CAD build for the part. Positions are in the model's coordinates, mm. Face numbers are marked on the shaded views. A direction names the side the tool comes from. Coordinates: 2 decimals unless noted, no trailing zeros. Order: outer loops, then holes, each group sorted by start corner. A loop starts at its lowest first (then second) coordinate and runs counter-clockwise, first axis right, second up. Notation, with made-up numbers: M 63,-36 L 118,-36 A20 ccw 118,-26 Z; hole C 70.5,30 d6. An arc over 180 degrees is marked long. One line per item, written item: value.
from build123d import *

# Parameters (mm, degrees)
SKETCH1_W           = 41.91
SKETCH1_H           = 41.91
SKETCH1_R           = 1.64973
SKETCH1_R_2         = 12.7
BOSS_EXTRUDE1_DEPTH = 10.795
SKETCH2_R           = 62.565718238
SKETCH2_R_2         = 27.7876
CUT_EXTRUDE1_DEPTH  = 61.244736077
SKETCH3_R           = 19.84375
CUT_EXTRUDE2_DEPTH  = 7.62


with BuildPart() as part:
    # Sketch1 → Boss-Extrude1 (new body)
    with BuildSketch(Plane.XY):
        with Locations((20.955, 20.955)):
            Rectangle(SKETCH1_W, SKETCH1_H)
        with Locations((37.460710751, 37.460710751)):
            Circle(SKETCH1_R, mode=Mode.SUBTRACT)
        with Locations((37.460710751, 4.449289249)):
            Circle(SKETCH1_R, mode=Mode.SUBTRACT)
        with Locations((4.449289249, 4.449289249)):
            Circle(SKETCH1_R, mode=Mode.SUBTRACT)
        with Locations((4.449289249, 37.460710751)):
            Circle(SKETCH1_R, mode=Mode.SUBTRACT)
        with Locations((20.955, 20.955)):
            Circle(SKETCH1_R_2, mode=Mode.SUBTRACT)
    extrude(amount=BOSS_EXTRUDE1_DEPTH)

    # Sketch2 → Cut-Extrude1 (cut, through all)
    with BuildSketch(Plane.XY.offset(10.795)):
        with Locations((20.955, 20.955)):
            Circle(SKETCH2_R)
        with Locations((20.955, 20.955)):
            Circle(SKETCH2_R_2, mode=Mode.SUBTRACT)
    extrude(amount=-CUT_EXTRUDE1_DEPTH, mode=Mode.SUBTRACT)

    # Sketch3 → Cut-Extrude2 (cut)
    with BuildSketch(Plane.XY.offset(10.795)):
        with Locations((20.955, 20.955)):
            Circle(SKETCH3_R)
    extrude(amount=-CUT_EXTRUDE2_DEPTH, mode=Mode.SUBTRACT)


solid = part.part
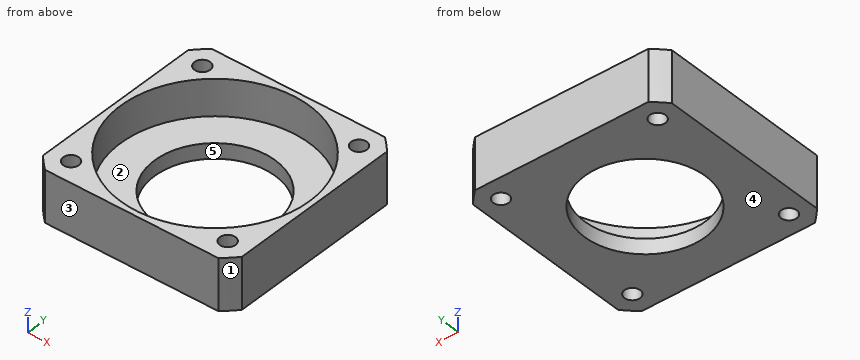
Q1. Drill centre lines: line 1 along Z through (x, y) = (32, 10.5) (3 decimals); line 2 along X through (y, z) = (30.5, 5); line 3 along X through (y, z) = (10, 4). Where is each one in solid material? Low to high.
Recorded:
line 1: z = 0 to 3.175
line 2: x = 0 to 3.56, 38.35 to 41.91
line 3: x = 0 to 4.41, 37.5 to 41.91
Q2. Mould opens along Y. For the marked faces 3, 4 and 5 say: released by +Y, released by -Y, zero draft, split by the parting line, or undercut.
Recorded:
face 3: released by -Y
face 4: zero draft
face 5: undercut
Q3. Slice it at B-B (x = 15.5). List the corners of the cut face in (y, z) (3 decimals), plus the area to 3 significant figures.
Recorded:
outline: M 0,0 L 9.486,0 L 9.486,3.175 L 1.876,3.175 L 1.876,10.795 L 0,10.795 Z; M 32.424,0 L 41.91,0 L 41.91,10.795 L 40.034,10.795 L 40.034,3.175 L 32.424,3.175 Z
area: 88.8 mm^2
Q4. Slice it at D-D (y = 5). List the corners of the cut face in (x, z) (3 decimals), plus the area to 3 significant figures.
Recorded:
outline: M 0,0 L 2.894,0 L 2.894,10.795 L 0,10.795 Z; M 6.004,0 L 35.906,0 L 35.906,10.795 L 32.754,10.795 L 32.754,3.175 L 9.156,3.175 L 9.156,10.795 L 6.004,10.795 Z; M 39.016,0 L 41.91,0 L 41.91,10.795 L 39.016,10.795 Z
area: 205 mm^2
Q5. Slice it at A-A (y = 24.5). List the corners of the cut face in (x, z) (3 decimals).
Recorded:
outline: M 0,0 L 8.76,0 L 8.76,3.175 L 1.43,3.175 L 1.43,10.795 L 0,10.795 Z; M 33.15,0 L 41.91,0 L 41.91,10.795 L 40.48,10.795 L 40.48,3.175 L 33.15,3.175 Z
Q6. Which spindle directions (+Z, -Z, +X, -X, +Y, -Y) get a long thin tool onto all of the face, cutting with end or side? Do the marked faces 1 and 2. Say none if no direction does.
Recorded:
face 1: +Z, -Z, +X, -Y
face 2: +Z
Q7. Pin check, flat tips, straight feed: pin 1 Ø5.5 at (x, y) = (37.46, 37.46) entering from +Z (3 decimals); pin 2 Ø20 at (x, y) = (27, 27.5) entering from +Z (3 decimals). Stop position of each tip, or through.
Recorded:
pin 1: stops at z = 10.795
pin 2: stops at z = 3.175
Q8. Slice it at C-C (z = 1.25). List the corners of the cut face in (x, y) (3 decimals).
Recorded:
outline: M 0,2.706 A27.788 ccw 2.706,0 L 39.204,0 A27.788 ccw 41.91,2.706 L 41.91,39.204 A27.788 ccw 39.204,41.91 L 2.706,41.91 A27.788 ccw 0,39.204 Z; hole C 4.449,4.449 d3.299; hole C 4.449,37.461 d3.299; hole C 20.955,20.955 d25.4; hole C 37.461,4.449 d3.299; hole C 37.461,37.461 d3.299
